from build123d import *

# Parameters (mm, degrees)
EXTRUDE_1_DEPTH     = 2.5
SKETCH_3_W          = 2.599185832
SKETCH_3_H          = 10
SKETCH_3_W_2        = 2.5
EXTRUDE_2_DEPTH     = 10
CUT_EXTRUDE_1_DEPTH = 59
SKETCH_5_R          = 1.75
CUT_EXTRUDE_2_DEPTH = 59
FILLET_1_R          = 1
SKETCH_6_R          = 1.75
CUT_EXTRUDE_3_DEPTH = 59


with BuildPart() as part:
    # 草图1 → 凸台-拉伸1 (new body)
    with BuildSketch(Plane(origin=(0, 0, 0), x_dir=(1, 0, 0), z_dir=(0, 1, 0))):
        with BuildLine():
            Line((-23, -5), (23, -5))
            ThreePointArc((23, -5), (24.414213562, -4.414213562), (25, -3))
            Line((25, -3), (25, 3))
            ThreePointArc((25, 3), (24.414213562, 4.414213562), (23, 5))
            Line((23, 5), (-23, 5))
            ThreePointArc((-23, 5), (-24.414213562, 4.414213562), (-25, 3))
            Line((-25, 3), (-25, -3))
            ThreePointArc((-25, -3), (-24.414213562, -4.414213562), (-23, -5))
        make_face()
    extrude(amount=EXTRUDE_1_DEPTH)

    # 草图3 → 凸台-拉伸2 (add)
    with BuildSketch(Plane(origin=(0, 2.5, 0), x_dir=(1, 0, 0), z_dir=(0, 1, 0))):
        with Locations((-21.700407084, 0)):
            Rectangle(SKETCH_3_W, SKETCH_3_H)
        with Locations((-13.150814168, 0)):
            Rectangle(SKETCH_3_W_2, SKETCH_3_H)
        with Locations((13.150814168, 0)):
            Rectangle(SKETCH_3_W_2, SKETCH_3_H)
        with Locations((21.700407084, 0)):
            Rectangle(SKETCH_3_W, SKETCH_3_H)
    extrude(amount=EXTRUDE_2_DEPTH)

    # 草图4 → 切除-拉伸1 (cut)
    with BuildSketch(Plane.ZY.offset(23)):
        Polygon((-2.5, 12.5), (-5, 5), (-5, 12.5), align=None)
        Polygon((5, 5), (5, 12.5), (2.5, 12.5), align=None)
    extrude(amount=-CUT_EXTRUDE_1_DEPTH, mode=Mode.SUBTRACT)

    # 草图5 → 切除-拉伸2 (cut)
    with BuildSketch(Plane.ZY.offset(23)):
        with Locations(Location((0, 8.5, 0), (0, 0, 180))):
            Circle(SKETCH_5_R)
    extrude(amount=-CUT_EXTRUDE_2_DEPTH, mode=Mode.SUBTRACT)

    # 圆角1
    fillet_1_edges = [part.edges().sort_by_distance(p)[0] for p in [
        (-13.150814168, 12.5, -2.5),
        (13.150814168, 12.5, -2.5),
        (-21.700407084, 12.5, -2.5),
        (-13.150814168, 12.5, 2.5),
        (13.150814168, 12.5, 2.5),
        (-21.700407084, 12.5, 2.5),
        (21.700407084, 12.5, 2.5),
        (21.700407084, 12.5, -2.5),
    ]]
    fillet(fillet_1_edges, radius=FILLET_1_R)

    # 草图6 → 切除-拉伸3 (cut)
    with BuildSketch(Plane(origin=(0, 2.5, 0), x_dir=(1, 0, 0), z_dir=(0, 1, 0))):
        with Locations(Location((-6.5, 0, 0), (0, 0, 270))):
            Circle(SKETCH_6_R)
        with Locations(Location((6.5, 0, 0), (0, 0, 270))):
            Circle(SKETCH_6_R)
    extrude(amount=-CUT_EXTRUDE_3_DEPTH, mode=Mode.SUBTRACT)


solid = part.part
Verification items for the finished model (mm, model axes). A direction names the side the tool comes from. Coordinates: 2 decimals unless noted, no trailing zeros. Write each loop counter-clockwise with the first axis right and the second up, starting at its lowest first coordinate (ties: lowest second). Pieces come first, ordered by that corner, then holes. Notation, with made-up numbers: M -12,-1.5 L 19,-1.5 A11 ccw 19,10.5 Z; hole C 85.5,37.25 d9. An arc over 180 degrees is marked long. Use a Markdown table: item, result.
Q1. Sectioned sample at D-D, the plane y = 9.5. Count the separate pieces of the cut face and the enclosed holes in it, plus the area to 3 significant figures.
Reply:
| item | result |
|---|---|
| separate pieces | 8 |
| enclosed holes | 0 |
| area | 42.1 mm² |
Q2. Set-up check for faces 4 (the face through (-20.401, 6, 0)), 5 (the face through (-23, 6, 0)), 6 (the face through (13.168, 12.306, -2.371)): record each of +Z, -Z, +X, -X, +Y, -Y from which the full face is reachable in a straight line by a thin tool's end or side.
Reply:
| item | result |
|---|---|
| face 4 | +Z, -Z, +Y |
| face 5 | +Z, -Z, -X, +Y |
| face 6 | -Z, +X, -X, +Y |
Q3. Draft check along X on faces 1 (the face through (-11.901, 6, 0)), 2 (the face through (24.4, 1.23, 4.43)), 3 (the face through (21.719, 12.306, -2.371)). Enter one of: +X half, -X half, draft (parallel to the pull), parting line (faces both ways), or undercut.
Reply:
| item | result |
|---|---|
| face 1 | undercut |
| face 2 | +X half |
| face 3 | draft |
Q4. Sectioned sample at A-A, the plane x = -6.5. Record the boundary of the cut face in (y, z), plus the area to 4 significant figures.
Reply:
| item | result |
|---|---|
| outline | M 0,-5 L 2.5,-5 L 2.5,-1.75 L 0,-1.75 Z; M 0,1.75 L 2.5,1.75 L 2.5,5 L 0,5 Z |
| area | 16.25 mm² |
Q5. Sectioned sample at B-B, the plane y = 1.5. Record the boundary of the cut face in (x, z).
Reply:
| item | result |
|---|---|
| outline | M -25,-3 A2 ccw -23,-5 L 23,-5 A2 ccw 25,-3 L 25,3 A2 ccw 23,5 L -23,5 A2 ccw -25,3 Z; hole C -6.5,0 d3.5; hole C 6.5,0 d3.5 |
Q6. Sectioned sample at C-C, the plane x = 22. Record the boundary of the cut face in (y, z), plus the area to 3 significant figures.
Reply:
| item | result |
|---|---|
| outline | M 0,-5 L 5,-5 L 11.82,-2.73 A1 ccw 12.5,-1.78 L 12.5,1.78 A1 ccw 11.82,2.73 L 5,5 L 0,5 Z; hole C 8.5,0 d3.5 |
| area | 96.4 mm² |
Q7. Thickness scan on line 1 (X direction, y = 3.5, z = 2.75); line 2 (Y direction, x = 12.7, z = 0); line 3 (Y direction, x = 11, z = -4.25). Record the ranges inside material, lowest first.
Reply:
| item | result |
|---|---|
| line 1 | x = -23 to -20.4, -14.4 to -11.9, 11.9 to 14.4, 20.4 to 23 |
| line 2 | y = 0 to 6.75, 10.25 to 12.5 |
| line 3 | y = 0 to 2.5 |
Q8. Go/stop test with flat-tipped pins: P1, Ø1.6, axis at x = -24.5, z = -1, coming from the +Y side; P2, Ø3, axis at y = 8.5, z = 0, coming from the -X side; P3, Ø1.5, axis at y = 4.5, z = -3, coming from the +X side; P4, Ø2, axis at y = 8, z = 3.5, coming from the -X side. Record where each tip stops, or that it passes through.
Reply:
| item | result |
|---|---|
| P1 | stops at y = 2.5 |
| P2 | passes through |
| P3 | stops at x = 23 |
| P4 | stops at x = -23 |
